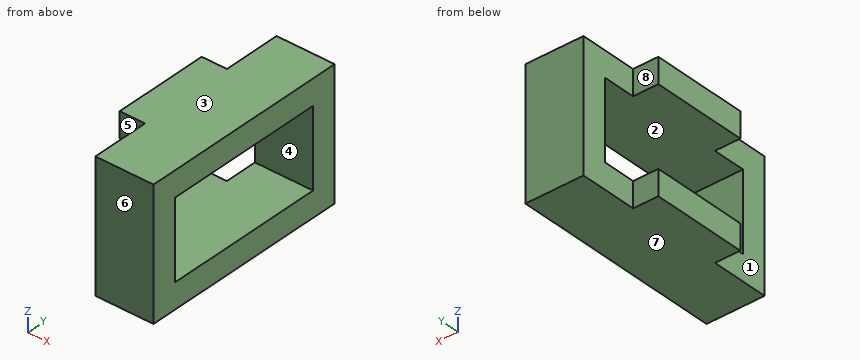
```python
from build123d import *

# Parameters (mm, degrees)
SKETCH063_W      = 2
SKETCH063_H      = 2
EXTRUDE068_DEPTH = 3.8
SKETCH062_W      = 4.6
SKETCH062_H      = 6.2
EXTRUDE067_DEPTH = 6.4
SKETCH061_W      = 4.6
SKETCH061_H      = 10.2
EXTRUDE066_DEPTH = 8.4


with BuildPart() as obj1:
    # Sketch063 → Extrude068 (new body, symmetric)
    with BuildSketch(Plane.XZ):
        with Locations((-3.3, 4.1)):
            Rectangle(SKETCH063_W, SKETCH063_H)
        with Locations((-3.3, -4.1)):
            Rectangle(SKETCH063_W, SKETCH063_H)
    extrude(amount=EXTRUDE068_DEPTH, both=True)


with BuildPart() as obj2:
    # Sketch062 → Extrude067 (new body, symmetric)
    with BuildSketch(Plane.XZ):
        Rectangle(SKETCH062_W, SKETCH062_H)
    extrude(amount=EXTRUDE067_DEPTH, both=True)


with BuildPart() as obj3:
    # Sketch061 → Extrude066 (new body, symmetric)
    with BuildSketch(Plane.XZ):
        Rectangle(SKETCH061_W, SKETCH061_H)
    extrude(amount=EXTRUDE066_DEPTH, both=True)

    # Cut036: cut obj2
    add(obj2.part, mode=Mode.SUBTRACT)

    # Fusion002: union obj1
    add(obj1.part)


solid = obj3.part
```
Geometry: final body of the model. Coordinates: model frame, mm. Face numbers are marked on the shaded views. A direction names the side the tool comes from. Coordinates: 2 decimals unless noted, no trailing zeros. Order: outer loops, then holes, each group sorted by start corner. A loop starts at its lowest first (then second) coordinate and runs counter-clockwise, first axis right, second up. Notation, with made-up numbers: (-17, 0.25) - (23, 0.25) arc R16 ccw to (23, 28.25) - close; hole circle Ø2 at (3, 5.5). An arc over 180 degrees is marked (long way). Return JSON: item names as keys, results as strings. Group by question number.
1. Cut plane D-D (z = -3.75). Output: boundary loops of the cut face in (x, y), plus the area to 3 significant figures.
2. Cut plane B-B (z = -1.25). Output: boundary loops of the cut face in (x, y), plus the area to 3 significant figures.
3. Pin query (flat end, axial travel): pin 1 (2.5 mm diameter, centred on y = -7, z = 2, fed in from -X); pin 2 (1 mm diameter, centred on x = -3.5, z = 3.5, fed in from -Y); pin 3 (1.5 mm diameter, centred on y = -4.5, z = -2, fed in from +X); pin 4 (1.6 mm diameter, centred on x = -3.5, z = 4, fed in from +Y). Return the tip coordinate at first contact, or that it passes through.
4. Cut plane C-C (x = 0). Output: boundary loops of the cut face in (y, z).
5. Cut plane A-A (y = -5.5). Output: boundary loops of the cut face in (x, z), plus the area to 3 significant figures.
6. Material intervals for line 1 along Z through (x, y) = (1, -0.75); line 2 along Y through (x, z) = (-1.5, -1); line 3 along X through (y, z) = (7.5, 1), sorted ascending. Write a range as [from, to].
7. Pull-direction query (Z, two-part tool) for the marked faces 1, 2 and 3; classes: pulls with the +Z half, pulls with the -Z half, needs draft (parallel to the pull), parting line crosses it, or undercut.
8. Set-up query: the marked faces 4, 5, 6, 7 and 8. Return all of +Z, -Z, +X, -X, +Y, -Y with unobstructed straight access to the full face (end or side cutting, diameter ignored); none if empty.
Resolved:
{
 "1": {"outline": "(-4.3, -3.8) - (-2.3, -3.8) - (-2.3, -8.4) - (2.3, -8.4) - (2.3, 8.4) - (-2.3, 8.4) - (-2.3, 3.8) - (-4.3, 3.8) - close", "area": "92.5 mm²"},
 "2": {"outline": "(-2.3, -8.4) - (2.3, -8.4) - (2.3, -6.4) - (-2.3, -6.4) - close; (-2.3, 6.4) - (2.3, 6.4) - (2.3, 8.4) - (-2.3, 8.4) - close", "area": "18.4 mm²"},
 "3": {"pin 1": "stops at x = -2.3", "pin 2": "stops at y = -3.8", "pin 3": "passes through", "pin 4": "stops at y = 3.8"},
 "4": {"outline": "(-8.4, -5.1) - (8.4, -5.1) - (8.4, 5.1) - (-8.4, 5.1) - close; hole (-6.4, -3.1) - (6.4, -3.1) - (6.4, 3.1) - (-6.4, 3.1) - close"},
 "5": {"outline": "(-2.3, -5.1) - (2.3, -5.1) - (2.3, -3.1) - (-2.3, -3.1) - close; (-2.3, 3.1) - (2.3, 3.1) - (2.3, 5.1) - (-2.3, 5.1) - close", "area": "18.4 mm²"},
 "6": {"line 1": "z = [-5.1, -3.1], [3.1, 5.1]", "line 2": "y = [-8.4, -6.4], [6.4, 8.4]", "line 3": "x = [-2.3, 2.3]"},
 "7": {"face 1": "needs draft", "face 2": "undercut", "face 3": "pulls with the +Z half"},
 "8": {"face 4": "+X, -X", "face 5": "+Z, -Z, -X, -Y", "face 6": "+Z, -Z, +X, -X, -Y", "face 7": "-Z, +X, -X, +Y, -Y", "face 8": "+Z, -Z, -X, +Y"}
}
